```python
from build123d import *

# Parameters (mm, degrees)
SKETCH1_R           = 8
BOSS_EXTRUDE1_DEPTH = 3.175


with BuildPart() as part:
    # Sketch1 → Boss-Extrude1 (new body)
    with BuildSketch(Plane(origin=(0, 0, 0), x_dir=(1, 0, 0), z_dir=(0, 1, 0))):
        Polygon((128.27, 0), (128.27, -3.175), (115.57, -3.175), (115.57, 0), (89.809134643, 0), (89.809134643, -3.175), (77.109134643, -3.175), (77.109134643, 0), (51.348269287, 0), (51.348269287, -3.175), (38.648269287, -3.175), (38.648269287, 0), (0, 0), (0, 63.5), (38.648269287, 63.5), (38.648269287, 66.675), (51.348269287, 66.675), (51.348269287, 63.5), (77.109134643, 63.5), (77.109134643, 66.675), (89.809134643, 66.675), (89.809134643, 63.5), (115.57, 63.5), (115.57, 66.675), (128.27, 66.675), (128.27, 63.5), (147.32, 63.5), (147.32, 0), align=None)
        with Locations(Location((25.4, 31.75, 0), (0, 0, 270))):
            Circle(SKETCH1_R, mode=Mode.SUBTRACT)
        Polygon((124.212866127, 50.8), (122.206447374, 38.259494277), (119.071320943, 38.761098966), (121.077739696, 51.301604688), align=None, mode=Mode.SUBTRACT)
        Polygon((117.064902189, 26.220593243), (115.058483436, 13.68008752), (118.193609867, 13.178482831), (120.20002862, 25.718988554), align=None, mode=Mode.SUBTRACT)
        Polygon((111.512866127, 50.8), (107.651646253, 38.701199188), (104.62694605, 39.666504157), (108.488165924, 51.765304968), align=None, mode=Mode.SUBTRACT)
        Polygon((100.765726177, 27.567703345), (96.904506303, 15.468902533), (99.929206506, 14.503597564), (103.79042638, 26.602398376), align=None, mode=Mode.SUBTRACT)
        Polygon((139.840468497, 20.301267714), (130.860212376, 11.321011593), (128.615148346, 13.566075623), (137.595404467, 22.546331745), align=None, mode=Mode.SUBTRACT)
        Polygon((69.226557851, 20.301267714), (57.802174059, 14.753885002), (56.415328381, 17.60998095), (67.839712173, 23.157363662), align=None, mode=Mode.SUBTRACT)
        Polygon((75.576557851, 28.17210754), (62.890656439, 27.573855616), (62.741093458, 30.745330969), (75.42699487, 31.343582893), align=None, mode=Mode.SUBTRACT)
    extrude(amount=BOSS_EXTRUDE1_DEPTH)


solid = part.part
```
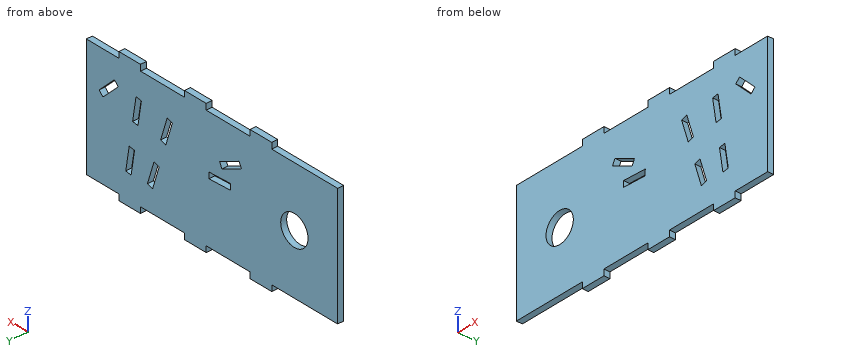
Work out the finished part from the listing and answer in its coordinate system (mm). Coordinates: 2 decimals unless noted, no trailing zeros. Loops run counter-clockwise (first coordinate to the right, second up) from the corner with the lowest first, then second, coordinate; pieces in that order, holes last. Notation, with made-up numbers: (-4, 25.25) - (17, 25.25) arc R13 ccw to (17, 37.25) - close; hole circle Ø4 at (85, 14). An arc over 180 degrees is marked (long way). Use a Markdown table: item, result.
Item 1: Find section C-C, the plane y = 0.85. State how many separate pieces and enclosed holes the cut face has, and give its area (3 significant figures).
Evaluation:
| item | result |
|---|---|
| separate pieces | 1 |
| enclosed holes | 8 |
| area | 9,110 mm2 |
Item 2: Find section B-B, the plane z = -48.5. Determine the outline of the cut face in (x, y) (1 decimal).
Evaluation:
| item | result |
|---|---|
| outline | (0, 0) - (107.4, 0) - (107.4, 3.2) - (0, 3.2) - close; (110.8, 0) - (120.6, 0) - (120.6, 3.2) - (110.8, 3.2) - close; (123.8, 0) - (147.3, 0) - (147.3, 3.2) - (123.8, 3.2) - close |
Item 3: Find section A-A, the plane x = 25.4. Determine the outline of the cut face in (y, z) (3 decimals).
Evaluation:
| item | result |
|---|---|
| outline | (0, -63.5) - (3.175, -63.5) - (3.175, -39.75) - (0, -39.75) - close; (0, -23.75) - (3.175, -23.75) - (3.175, 0) - (0, 0) - close |
Item 4: Consider probe 1 along X at (y, z) = (0.8, -31.75); probe 2 along X at (y, z) = (0.65, -25.5) (3 decimals); probe 3 along X at (y, z) = (2.65, -19.5). Determine where each line is inside the solid, lowest interval first. Write a range as from..to.
Evaluation:
| item | result |
|---|---|
| probe 1 | x = 0..17.4, 33.4..147.32 |
| probe 2 | x = 0..20.406, 30.394..100.106, 103.439..116.95, 120.165..147.32 |
| probe 3 | x = 0..60.31, 67.58..98.19, 101.52..115.99, 119.21..134.55, 139.04..147.32 |
Item 5: Given pin 1 Ø1 at (x, y) = (140, 2) entering from -Z; pin 2 Ø1.6 at (y, z) = (2.5, 2.5) entering from -X; pin 3 Ø1.6 at (y, z) = (1, 2) entering from +X, each flat-ended and moving along its own axis, determine where each tip first touches the part or whether it passes through.
Evaluation:
| item | result |
|---|---|
| pin 1 | stops at z = -63.5 |
| pin 2 | stops at x = 38.65 |
| pin 3 | stops at x = 128.27 |
